The model under review builds one solid part; all positions refer to its coordinate system, in mm. Face numbers are marked on the shaded views. A direction names the side the tool comes from. Coordinates: 2 decimals unless noted, no trailing zeros. Write each loop counter-clockwise with the first axis right and the second up, starting at its lowest first coordinate (ties: lowest second). Pieces come first, ordered by that corner, then holes. Notation, with made-up numbers: M 8.25,27 L 52.25,27 A13 ccw 52.25,32 Z; hole C 53.5,65 d6. An arc over 180 degrees is marked long. Answer as a JSON object with one key per item and string values.
```python
from build123d import *

# Parameters (mm, degrees)
SKETCH1_W               = 20
SKETCH1_H               = 90
BOSS_EXTRUDE1_DEPTH     = 20
CUT_EXTRUDE1_REACH      = 22
SKETCH2_W               = 15
SKETCH2_H               = 86
SKETCH3_R               = 2
CUT_EXTRUDE2_DEPTH      = 1
CUT_EXTRUDE2_DEPTH_BACK = 140


with BuildPart() as part:
    # Sketch1 → Boss-Extrude1 (new body)
    with BuildSketch(Plane.XY):
        Rectangle(SKETCH1_W, SKETCH1_H)
    extrude(amount=BOSS_EXTRUDE1_DEPTH)

    # Sketch2 → Cut-Extrude1 (cut, up to next)
    with BuildSketch(Plane(origin=(10, 0, 0), x_dir=(0, 0, -1), z_dir=(1, 0, 0)), mode=Mode.PRIVATE) as cut_extrude1_sk1:
        with Locations((-12.5, 0)):
            Rectangle(SKETCH2_W, SKETCH2_H)
    cut_extrude1_tool1 = extrude(cut_extrude1_sk1.sketch, amount=-CUT_EXTRUDE1_REACH, mode=Mode.PRIVATE) & part.part
    add(cut_extrude1_tool1.solids().sort_by_distance((10, 0, 12.5))[0], mode=Mode.SUBTRACT)

    # Sketch3 → Cut-Extrude2 (cut, two sides)
    with BuildSketch(Plane(origin=(0, 45, 0), x_dir=(1, 0, 0), z_dir=(0, 1, 0))) as cut_extrude2_sk:
        with Locations((-5, -12.5)):
            Circle(SKETCH3_R)
        with Locations((5, -12.5)):
            Circle(SKETCH3_R)
    extrude(amount=CUT_EXTRUDE2_DEPTH, mode=Mode.SUBTRACT)
    extrude(cut_extrude2_sk.sketch, amount=-CUT_EXTRUDE2_DEPTH_BACK, mode=Mode.SUBTRACT)


solid = part.part
```
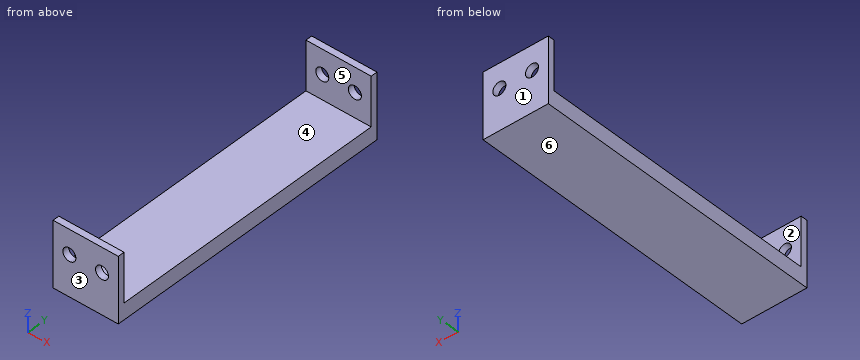
(1) Draft analysis for pull direction Y (two halves, no side actions). For the marked faces 3, 4, 5 and 6, state which applies: released by +Y, released by -Y, zero draft, split by the parting line, or undercut.
Results list:
{"face 3": "released by -Y", "face 4": "undercut", "face 5": "undercut", "face 6": "zero draft"}
(2) Add section D-D on y = 35. Give the boundary of the cut face in (x, z), and give its area (3 significant figures).
Results list:
{"outline": "M -10,0 L 10,0 L 10,5 L -10,5 Z", "area": "100 mm²"}
(3) Wall thickness on line 1 along X through (y, z) = (-44.3, 12.5); line 2 along Y through (x, z) = (-5.5, 8.75); line 3 along Z through (x, y) = (5, 43.9): over which ranges is each line inside the solid? List them lowest first. Write a range as from..to.
Results list:
{"line 1": "-10..-7, -3..3, 7..10", "line 2": "-45..-43, 43..45", "line 3": "0..10.5, 14.5..20"}
(4) Add section B-B on z = 12.5. Give the boundary of the cut face in (x, y), and give its area (3 significant figures).
Results list:
{"outline": "M -10,-45 L -7,-45 L -7,-43 L -10,-43 Z; M -10,43 L -7,43 L -7,45 L -10,45 Z; M -3,-45 L 3,-45 L 3,-43 L -3,-43 Z; M -3,43 L 3,43 L 3,45 L -3,45 Z; M 7,-45 L 10,-45 L 10,-43 L 7,-43 Z; M 7,43 L 10,43 L 10,45 L 7,45 Z", "area": "48.0 mm²"}
(5) For the marked faces 1 and 2, list the 3-axis set-ups (+Z, -Z, +X, -X, +Y, -Y) from which the entire face can be reached by the end or side of a thin tool; tool diameter is ignored.
Results list:
{"face 1": "+Z, -Z, +X, -X, +Y", "face 2": "+Z, +X, -X"}
(6) Add section C-C on x = 8. Give the boundary of the cut face in (y, z).
Results list:
{"outline": "M -45,0 L 45,0 L 45,20 L 43,20 L 43,5 L -43,5 L -43,20 L -45,20 Z"}
(7) Add section A-A on x = -5. Give the boundary of the cut face in (y, z), and give its area (3 significant figures).
Results list:
{"outline": "M -45,0 L 45,0 L 45,10.5 L 43,10.5 L 43,5 L -43,5 L -43,10.5 L -45,10.5 Z; M -45,14.5 L -43,14.5 L -43,20 L -45,20 Z; M 43,14.5 L 45,14.5 L 45,20 L 43,20 Z", "area": "494 mm²"}
(8) For pin 1 Ø2 at (x, y) = (7.5, -32.5) entering from +Z; pin 2 Ø4.5 at (x, z) = (5, 12.5) entering from +Y, all flat-tipped, find the tip position at first contact; note any pin that passes through.
Results list:
{"pin 1": "z = 5", "pin 2": "y = 45"}
